from build123d import *

# Parameters (mm, degrees)
MAIN_DEPTH          = 10
SKETCH1_W           = 26.5
SKETCH1_H           = 18
CUT_EXTRUDE1_DEPTH  = 7.5
ESQUISSE2_R         = 2.5
BOSS_EXTRUDE1_DEPTH = 2


with BuildPart() as part:
    # Esquisse1 → Main (new body)
    with BuildSketch(Plane.XY):
        with BuildLine():
            Line((-4.375785644, 4.25), (-6.426543071, 6.300757427))
            ThreePointArc((-6.426543071, 6.300757427), (-3.48519606, 8.297795395), (0, 9))
            Line((0, 9), (41, 9))
            ThreePointArc((41, 9), (50, 0), (41, -9))
            Line((41, -9), (0, -9))
            ThreePointArc((0, -9), (-3.48519606, -8.297795395), (-6.426543071, -6.300757427))
            Line((-6.426543071, -6.300757427), (-4.375785644, -4.25))
            ThreePointArc((-4.375785644, -4.25), (0, -6.1), (4.375785644, -4.25))
            Line((4.375785644, -4.25), (17.31559729, -2.78215714))
            ThreePointArc((17.31559729, -2.78215714), (19.8, 0), (17.31559729, 2.78215714))
            Line((17.31559729, 2.78215714), (4.375785644, 4.25))
            ThreePointArc((4.375785644, 4.25), (0, 6.1), (-4.375785644, 4.25))
        make_face()
        with BuildLine():
            Line((26, 5.25), (41, 5.25))
            ThreePointArc((41, 5.25), (46.25, 0), (41, -5.25))
            Line((41, -5.25), (26, -5.25))
            ThreePointArc((26, -5.25), (20.75, 0), (26, 5.25))
        make_face(mode=Mode.SUBTRACT)
    extrude(amount=MAIN_DEPTH)

    # Sketch1 → Cut-Extrude1 (cut)
    with BuildSketch(Plane.XY.offset(10)):
        with Locations((6.823456929, 0)):
            Rectangle(SKETCH1_W, SKETCH1_H)
    extrude(amount=-CUT_EXTRUDE1_DEPTH, mode=Mode.SUBTRACT)

    # Esquisse2 → Boss-Extrude1 (add)
    with BuildSketch(Plane(origin=(0, 0, 2.5), x_dir=(-1, 0, 0), z_dir=(0, 0, -1))):
        with BuildLine():
            Line((0, -9), (-20.073456929, -9))
            Line((-20.073456929, -9), (-20.073456929, 9))
            Line((-20.073456929, 9), (0, 9))
            ThreePointArc((0, 9), (3.48519606, 8.297795395), (6.426543071, 6.300757427))
            Line((6.426543071, 6.300757427), (6.426543071, -6.300757427))
            ThreePointArc((6.426543071, -6.300757427), (3.48519606, -8.297795395), (0, -9))
        make_face()
        Circle(ESQUISSE2_R, mode=Mode.SUBTRACT)
    extrude(amount=-BOSS_EXTRUDE1_DEPTH)


solid = part.part
Geometry check sheet. Reference: the model listing, model coordinates, mm. A direction names the side the tool comes from. Round coordinates to 2 decimals unless told otherwise and drop trailing zeros. Order: outer loops, then holes, each group sorted by start corner. A loop starts at its lowest first (then second) coordinate and runs counter-clockwise, first axis right, second up. Notation, with made-up numbers: (60.5, 84) -> (103.5, 84) arc R11 ccw to (103.5, 94) -> close; hole circle Ø5 at (42.25, 67). An arc over 180 degrees is marked (long way). Use one line per item in the form item = value.
1. Set-up check for faces 1 (the face through (34, -5.25, 5)), 2 (the face through (0.1, 6.1, 1.2)), 3 (the face through (-5.387, 5.261, 1.232)): record each of +Z, -Z, +X, -X, +Y, -Y from which the full face is reachable in a straight line by a thin tool's end or side.
Working result:
face_1 = +Z, -Z
face_2 = -Z
face_3 = -Z, -X
2. Scan lines: line 1 along Y through (x, z) = (0, 3.55); line 2 along Y through (x, z) = (31, 5.5); line 3 along X through (y, z) = (-0.25, 6). Record each from-to range of solid material in increasing order. Write a range as from..to.
Working result:
line_1 = -9..-2.5, 2.5..9
line_2 = -9..-5.25, 5.25..9
line_3 = 20.07..20.76, 46.24..50
3. Cross-section at A-A, the plane z = 1. Enter the section's corners in (x, y).
Working result:
outline = (-6.43, -6.3) arc R9 ccw to (0, -9) -> (41, -9) arc R9 ccw to (41, 9) -> (0, 9) arc R9 ccw to (-6.43, 6.3) -> (-4.38, 4.25) arc R6.1 cw to (4.38, 4.25) -> (17.32, 2.78) arc R2.8 cw to (17.32, -2.78) -> (4.38, -4.25) arc R6.1 cw to (-4.38, -4.25) -> close; hole (26, -5.25) -> (41, -5.25) arc R5.25 ccw to (41, 5.25) -> (26, 5.25) arc R5.25 ccw to start
4. Cross-section at C-C, the plane x = 37.5. Enter the section's corners in (y, z).
Working result:
outline = (-9, 0) -> (-5.25, 0) -> (-5.25, 10) -> (-9, 10) -> close; (5.25, 0) -> (9, 0) -> (9, 10) -> (5.25, 10) -> close
5. Cross-section at B-B, the plane y = 0. Enter the section's corners in (x, z), plus the area to 3 significant figures.
Working result:
outline = (-6.43, 2.5) -> (-2.5, 2.5) -> (-2.5, 4.5) -> (-6.43, 4.5) -> close; (2.5, 2.5) -> (19.8, 2.5) -> (19.8, 0) -> (20.75, 0) -> (20.75, 10) -> (20.07, 10) -> (20.07, 4.5) -> (2.5, 4.5) -> close; (46.25, 0) -> (50, 0) -> (50, 10) -> (46.25, 10) -> close
area = 87.9 mm^2
6. Mould release check, pull along Y, two halves, no side actions. Record for faces 4 (the face through (25, -9, 4)), 5 (the face through (7, 0, 4.5)), 6 (the face through (19.8, -0.1, 1.2)): pulls with the +Y half, pulls with the -Y half, needs draft (parallel to the pull), parting line crosses it, or undercut.
Working result:
face_4 = pulls with the -Y half
face_5 = needs draft
face_6 = undercut
7. Cross-section at D-D, the plane y = 3.75. Enter the section's corners in (x, z).
Working result:
outline = (-6.43, 2.5) -> (8.78, 2.5) -> (8.78, 0) -> (22.33, 0) -> (22.33, 10) -> (20.07, 10) -> (20.07, 4.5) -> (-6.43, 4.5) -> close; (44.67, 0) -> (49.18, 0) -> (49.18, 10) -> (44.67, 10) -> close
8. Go/stop test with flat-tipped pins: pin 1 (9 mm diameter, centred on x = 5, y = 0, fed in from +Z); pin 2 (4.5 mm diameter, centred on y = -2.5, z = 7, fed in from -X). Record where each tip stops, or that it passes through.
Working result:
pin_1 = 4.5
pin_2 = 20.07
